from build123d import *

# Parameters (mm, degrees)
F0_W     = 77.8246372938
F0_H     = 112.5469133258
F0_W_2   = 21.9748611562
F0_H_2   = 3.6779557122
F0_W_3   = 22.0251933206
F1_DEPTH = 7.366
F2_R     = 7.9006710882
F2_R_2   = 9.1916040088
F2_R_3   = 9.0636867771
F2_R_4   = 8.7975277967
F2_R_5   = 9.2142672279
F3_DEPTH = 79.248
F4_R     = 0.8182750857
F4_R_2   = 0.8655541006
F5_DEPTH = 7.8486
F7_START = 7.7978
F6_R     = 40.6030276707
F6_R_2   = 27.6936887415
F7_DEPTH = 7.6962
F9_START = 72.898
F8_W     = 76.8951624632
F8_H     = 111.9272559881
F8_W_2   = 56.9818727672
F8_H_2   = 37.3910360504
F9_DEPTH = 12.446


with BuildPart() as f1:
    # F0 (on Front) → F1 (new body)
    with BuildSketch(Plane.XZ):
        Rectangle(F0_W, F0_H)
        Polygon((-2.5131949224, -39.1017198563), (-24.4880560786, -39.1017198563), (-24.4880560786, -1.622540527), (-24.4880560786, 2.0554151852), (-24.4880560786, 39.1017198563), (-2.5131949224, 39.1017198563), (2.462862758, 39.1017198563), (24.4880560786, 39.1017198563), (24.4880560786, 2.0554151852), (24.4880560786, -1.622540527), (24.4880560786, -39.1017198563), (2.462862758, -39.1017198563), align=None, mode=Mode.SUBTRACT)
        with Locations((-13.5006255005, 0.2164373291)):
            Rectangle(F0_W_2, F0_H_2)
        with Locations((13.4754594183, 0.2164373291)):
            Rectangle(F0_W_3, F0_H_2)
        Polygon((-2.5131949224, -1.622540527), (-2.5131949224, -39.1017198563), (2.462862758, -39.1017198563), (2.462862758, -1.622540527), (2.462862758, 2.0554151852), (2.462862758, 39.1017198563), (-2.5131949224, 39.1017198563), (-2.5131949224, 2.0554151852), align=None)
    extrude(amount=F1_DEPTH)

    # F2 (on Front) → F3 (join)
    with BuildSketch(Plane.XZ):
        Circle(F2_R)
        with Locations((31.2162749469, 46.9267778099)):
            Circle(F2_R_2)
        with Locations((-28.8526788354, 48.0819493532)):
            Circle(F2_R_3)
        with Locations((30.9274848551, -45.1982095838)):
            Circle(F2_R_4)
        with Locations((-29.4302646071, -45.4870015383)):
            Circle(F2_R_5)
    extrude(amount=F3_DEPTH)

    # F4 (on Front) → F5 (join)
    with BuildSketch(Plane.XZ):
        with Locations((33.0372042954, 0)):
            Circle(F4_R)
        with Locations((-32.0478864014, 0)):
            Circle(F4_R_2)
    extrude(amount=F5_DEPTH)

    # F6 (on Front) → F7 (join)
    with BuildSketch(Plane.XZ.offset(F7_START)):
        Circle(F6_R)
        Circle(F6_R_2, mode=Mode.SUBTRACT)
    extrude(amount=F7_DEPTH)

    # F8 (on Front) → F9 (join)
    with BuildSketch(Plane.XZ.offset(F9_START)):
        Rectangle(F8_W, F8_H)
        with Locations((0, -22.4545601523)):
            Rectangle(F8_W_2, F8_H_2, mode=Mode.SUBTRACT)
        with Locations((0, 22.4545601523)):
            Rectangle(F8_W_2, F8_H_2, mode=Mode.SUBTRACT)
    extrude(amount=F9_DEPTH)


solid = f1.part
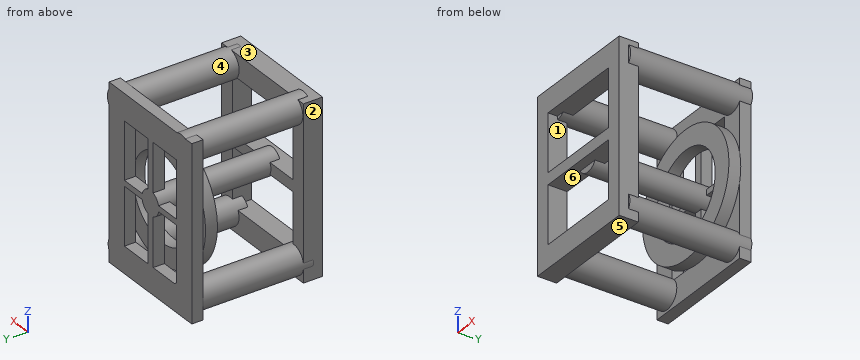
Input: part model. Units: mm. Frame: model coordinates. Face numbers are marked on the shaded views. A direction names the side the tool comes from. Round coordinates to 2 decimals unless told otherwise and drop trailing zeros. Loops run counter-clockwise (first coordinate to the right, second up) from the corner with the lowest first, then second, coordinate; pieces in that order, holes last. Notation, with made-up numbers: M -15.5,46.25 L 37.5,46.25 A25 ccw 37.5,71.25 Z; hole C -26.5,79.5 d3. An arc over 180 degrees is marked long. Answer as CSV lines item,"result". Start each with the question number.
(1) First-contact query: pin 1 (1 mm diameter, centred on x = 39.5, z = 49, fed in from -Y); pin 2 (4 mm diameter, centred on y = -76.5, z = 6, fed in from +X); pin 3 (4.5 mm diameter, centred on x = -5.5, z = -48, fed in from +Y); pin 4 (1 mm diameter, centred on x = 20, y = -42.5, fed in from -Z). Flat tips, straight axial feed; report the tip coordinate or a pass-through.
(2) Line query: line 1 (Z direction, x = 0, y = -10); line 2 (Z direction, x = -28, y = -79.5); line 3 (Y direction, x = 36, z = -15.5). Output: solid intervals per line, ascending. Write a range as [from, to].
(3) Section C-C, the plane z = 19. Output: boundary loops of the cut face in (x, y).
(4) Reachability of the marked faces 4, 5 and 6 from +Z, -Z, +X, -X, +Y, -Y: full face, straight path, thin tool, end or side. Return the list, or none.
(5) Section D-D, the plane x = -18. State how many separate pieces and enclosed holes the cut face has, plus the area to 3 significant figures.
(6) Section B-B, the plane y = -10. Output: boundary loops of the cut face in (x, z), plus the area to 3 significant figures.
(7) Draft query along Z for the marked faces 1, 2 and 3. Return one class per face: released by +Z, released by -Z, zero draft, split by the parting line, or undercut.
(8) Section A-A, the plane x = 0. Output: boundary loops of the cut face in (y, z), plus the area to 3 significant figures.
Values found:
1,pin 1,"stops at y = -79.25"
1,pin 2,"stops at x = 38.45"
1,pin 3,"stops at y = 0"
1,pin 4,"passes through"
2,line 1,"z = [-40.6, -27.69], [-7.9, 7.9], [27.69, 40.6]"
2,line 2,"z = [-55.96, -41.15], [-3.76, 3.76], [41.15, 55.96]"
2,line 3,"y = [-85.34, -72.9], [-15.49, -7.8], [-7.37, 0]"
3,outline,"M -38.91,-7.37 L -24.49,-7.37 L -24.49,0 L -38.91,0 Z; M -38.45,-85.34 L -28.49,-85.34 L -28.49,-72.9 L -38.45,-72.9 Z; M -35.88,-15.49 L -20.15,-15.49 L -20.15,-7.8 L -35.88,-7.8 Z; M -2.51,-7.37 L 2.46,-7.37 L 2.46,0 L -2.51,0 Z; M 20.15,-15.49 L 35.88,-15.49 L 35.88,-7.8 L 20.15,-7.8 Z; M 24.49,-7.37 L 38.91,-7.37 L 38.91,0 L 24.49,0 Z; M 28.49,-85.34 L 38.45,-85.34 L 38.45,-72.9 L 28.49,-72.9 Z"
4,face 4,"none"
4,face 5,"-Z, +X, -X, -Y"
4,face 6,"-Y"
5,separate pieces,"8"
5,enclosed holes,"0"
5,area,"979 mm²"
6,outline,"C 0,0 d81.21; C -29.43,-45.49 d18.43; C -28.85,48.08 d18.13; C 0,0 d15.8; C 31.22,46.93 d18.38; C 30.93,-45.2 d17.6; hole C 0,0 d55.39"
6,area,"4,000 mm²"
7,face 1,"undercut"
7,face 2,"zero draft"
7,face 3,"released by +Z"
8,outline,"M -85.34,-55.96 L -72.9,-55.96 L -72.9,-41.15 L -85.34,-41.15 Z; M -85.34,-3.76 L -79.25,-3.76 L -79.25,-7.9 L -7.37,-7.9 L -7.37,-56.27 L 0,-56.27 L 0,56.27 L -7.37,56.27 L -7.37,7.9 L -79.25,7.9 L -79.25,3.76 L -85.34,3.76 Z; M -85.34,41.15 L -72.9,41.15 L -72.9,55.96 L -85.34,55.96 Z; M -15.49,-40.6 L -7.8,-40.6 L -7.8,-27.69 L -15.49,-27.69 Z; M -15.49,27.69 L -7.8,27.69 L -7.8,40.6 L -15.49,40.6 Z"
8,area,"2,580 mm²"
